Read the model definition and answer for the solid it produces. Units are mm, in the model's axes. A direction names the side the tool comes from. Coordinates: 2 decimals unless noted, no trailing zeros. Write each loop counter-clockwise with the first axis right and the second up, starting at its lowest first coordinate (ties: lowest second). Pieces come first, ordered by that corner, then holes. Notation, with made-up numbers: M 38.25,-21.5 L 60.25,-21.5 A25 ccw 60.25,9.5 Z; hole C 89,15.25 d11. An arc over 180 degrees is marked long. Write item = value, one per line.
from build123d import *

# Parameters (mm, degrees)
SKETCH1_W           = 88.9
SKETCH1_H           = 12.7
SKETCH1_R           = 2.54
BOSS_EXTRUDE2_DEPTH = 5.08
SKETCH2_R           = 2.794
BOSS_EXTRUDE3_DEPTH = 5.08
FILLET1_R           = 1.27
SKETCH3_R           = 4.7625
CUT_EXTRUDE1_DEPTH  = 2.54


with BuildPart() as part:
    # Sketch1 → Boss-Extrude2 (new body)
    with BuildSketch(Plane(origin=(0, 0, 0), x_dir=(1, 0, 0), z_dir=(0, 1, 0))):
        with Locations((44.45, 6.35)):
            Rectangle(SKETCH1_W, SKETCH1_H)
        with Locations(Location((34.925, 6.35, 0), (0, 0, 270))):
            Circle(SKETCH1_R, mode=Mode.SUBTRACT)
        with Locations(Location((53.975, 6.35, 0), (0, 0, 270))):
            Circle(SKETCH1_R, mode=Mode.SUBTRACT)
    extrude(amount=BOSS_EXTRUDE2_DEPTH)

    # Sketch2 → Boss-Extrude3 (add)
    with BuildSketch(Plane(origin=(0, 5.08, 0), x_dir=(1, 0, 0), z_dir=(0, 1, 0))):
        with Locations(Location((19.05, 6.35, 0), (0, 0, 270))):
            Circle(SKETCH2_R)
        with Locations(Location((69.85, 6.35, 0), (0, 0, 90))):
            Circle(SKETCH2_R)
    extrude(amount=BOSS_EXTRUDE3_DEPTH)

    # Fillet1
    fillet1_edges = [part.edges().sort_by_distance(p)[0] for p in [
        (19.05, 10.16, -9.144),
        (69.85, 10.16, -3.556),
    ]]
    fillet(fillet1_edges, radius=FILLET1_R)

    # Sketch3 → Cut-Extrude1 (cut)
    with BuildSketch(Plane(origin=(0, 5.08, 0), x_dir=(1, 0, 0), z_dir=(0, 1, 0))):
        with Locations(Location((34.925, 6.35, 0), (0, 0, 270))):
            Circle(SKETCH3_R)
        with Locations(Location((53.975, 6.35, 0), (0, 0, 270))):
            Circle(SKETCH3_R)
    extrude(amount=-CUT_EXTRUDE1_DEPTH, mode=Mode.SUBTRACT)


solid = part.part
Item 1: Consider line 1 along X through (y, z) = (2, -6.35) (3 decimals); line 2 along X through (y, z) = (5.75, -4); line 3 along X through (y, z) = (4.4, -6.35). Determine where each line is inside the solid, lowest interval first. Write a range as from..to.
Worked answers:
line_1 = 0..32.385, 37.465..51.435, 56.515..88.9
line_2 = 17.54..20.56, 68.34..71.36
line_3 = 0..30.16, 39.69..49.21, 58.74..88.9
Item 2: For a pull along Z with two mould halves and no side action, classify faces 3 (the face through (0, 3, -6)), 4 (the face through (39.647, 3.828, -6.97)), 5 (the face through (44, 3, -12.7)) as released by +Z, released by -Z, zero draft, split by the parting line, or undercut.
Worked answers:
face_3 = zero draft
face_4 = undercut
face_5 = released by -Z
Item 3: Which of the six approach directions +Z, -Z, +X, -X, +Y, -Y give full straight-line access (tool end or side, diameter ignored) to faces 1 (the face through (70, 10.16, -6)), 2 (the face through (49.326, 3.828, -7.382))?
Worked answers:
face_1 = +Z, -Z, +X, -X, +Y
face_2 = +Y
Item 4: Flat-ended cylindrical pins translate along their axes: pin 1 (2 mm diameter, centred on y = 3, z = -4, fed in from -X); pin 2 (2 mm diameter, centred on y = 9, z = -8.5, fed in from +X); pin 3 (5 mm diameter, centred on x = 29.5, z = -11, fed in from +Y). Find the tip coordinate at first contact, or state that the pin passes through.
Worked answers:
pin_1 = 0
pin_2 = 72.39
pin_3 = 5.08
Item 5: Find section D-D (y = 1.25). Determine the outline of the cut face in (x, z) (3 decimals).
Worked answers:
outline = M 0,-12.7 L 88.9,-12.7 L 88.9,0 L 0,0 Z; hole C 34.925,-6.35 d5.08; hole C 53.975,-6.35 d5.08
Item 6: Find section C-C (y = 6.25). Determine the outline of the cut face in (x, z), and give its area (3 significant figures).
Worked answers:
outline = C 19.05,-6.35 d5.59; C 69.85,-6.35 d5.59
area = 49.0 mm²
Item 7: Find section A-A (z = -6.35). State how many separate pieces and enclosed holes the cut face has, and give its area (3 significant figures).
Worked answers:
separate_pieces = 3
enclosed_holes = 0
area = 433 mm²
Item 8: Find section B-B (x = 19.05). Determine the outline of the cut face in (y, z), and give its area (3 significant figures).
Worked answers:
outline = M 0,-12.7 L 5.08,-12.7 L 5.08,-9.14 L 8.89,-9.14 A1.27 ccw 10.16,-7.87 L 10.16,-4.83 A1.27 ccw 8.89,-3.56 L 5.08,-3.56 L 5.08,0 L 0,0 Z
area = 92.2 mm²
